The figure shows three views and two pictorial views of one solid part (mm, origin at its lowest corner). Answer the questions. A direction names the side the tool comes from. Give positions to 0.01 mm unless a question says otherwise; leave off trailing zeros. Loops run counter-clockwise (first coordinate to the right, second up) from the corner with the lowest first, then second, coordinate; pieces in that order, holes last. Notation, with made-up numbers: (79.5, 73.25) - (126.5, 73.25) arc R24 cw to (126.5, 95.25) - close; hole circle Ø7 at (47.5, 32). An arc over 180 degrees is marked (long way). Write item = value, one per line.
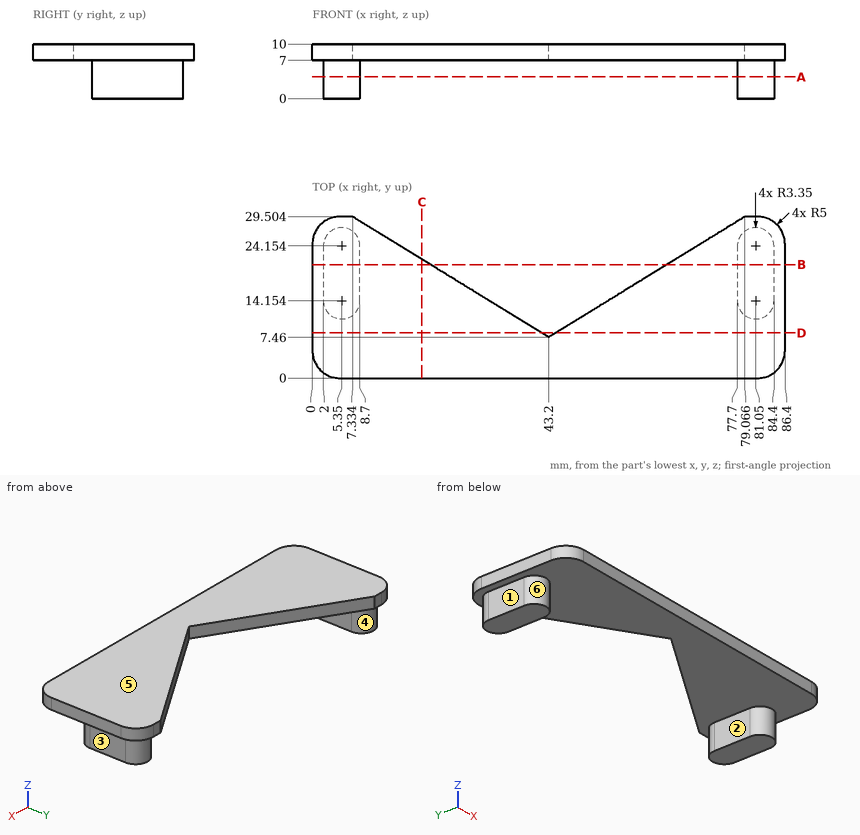
1) A cutting plane is placed at A-A on z = 4. Determine the outline of the cut face in (x, y).
Output:
outline = (2, 14.15) arc R3.35 ccw to (8.7, 14.15) - (8.7, 24.15) arc R3.35 ccw to (2, 24.15) - close; (77.7, 14.15) arc R3.35 ccw to (84.4, 14.15) - (84.4, 24.15) arc R3.35 ccw to (77.7, 24.15) - close
2) A cutting plane is placed at B-B on y = 20.75. Determine the outline of the cut face in (x, z).
Output:
outline = (0, 7) - (2, 7) - (2, 0) - (8.7, 0) - (8.7, 7) - (21.58, 7) - (21.58, 10) - (0, 10) - close; (64.82, 7) - (77.7, 7) - (77.7, 0) - (84.4, 0) - (84.4, 7) - (86.4, 7) - (86.4, 10) - (64.82, 10) - close
3) A cutting plane is placed at C-C on x = 20. Determine the outline of the cut face in (y, z).
Output:
outline = (0, 7) - (21.72, 7) - (21.72, 10) - (0, 10) - close
4) Find the intervals of material crossed by probe 1 along X at (y, z) = (22.25, 4.25); probe 2 along Z at (x, y) = (18.5, 2.5); probe 3 along X at (y, z) = (25.25, 2.75) (1 decimal), in increasing order.
Output:
probe_1 = 2 to 8.7, 77.7 to 84.4
probe_2 = 7 to 10
probe_3 = 2.2 to 8.5, 77.9 to 84.2
5) A tool of negligible diameter and unlimited length cuts with its end or side. For the marked faces 4, 5 and 6, from which of +Z, -Z, +X, -X, +Y, -Y can it reach the whole face along a straight path? Write none if from no direction.
Output:
face_4 = -Z, +Y
face_5 = +Z, +X, -X, +Y, -Y
face_6 = -Z, -Y
6) A cutting plane is placed at D-D on y = 8.25. Determine the outline of the cut face in (x, z) (1 decimal).
Output:
outline = (0, 7) - (41.9, 7) - (41.9, 10) - (0, 10) - close; (44.5, 7) - (86.4, 7) - (86.4, 10) - (44.5, 10) - close
7) The mould has two halves that part along X. Classify the marked faces 1, 2 and 3: pulls with the +X half, pulls with the -X half, needs draft (parallel to the pull), parting line crosses it, or undercut.
Output:
face_1 = pulls with the -X half
face_2 = undercut
face_3 = pulls with the +X half
8) Each of these flat-tipped pins is pushed along its axis until it touches: P1, Ø2, axis at y = 19, z = 2.5, coming from the +X side; P2, Ø6, axis at x = 41, y = 5, coming from the -Z side; P3, Ø3.5, axis at y = 18, z = 3, coming from the -X side. Where does it stop, or does it pass through?
Output:
P1 = 84.4
P2 = 7
P3 = 2
